The model under review builds one solid part; all positions refer to its coordinate system, in mm. A direction names the side the tool comes from. Coordinates: 2 decimals unless noted, no trailing zeros. Loops run counter-clockwise (first coordinate to the right, second up) from the corner with the lowest first, then second, coordinate; pieces in that order, holes last. Notation, with made-up numbers: M -15,79 L 0,79 A20 ccw 0,107 Z; hole C 27.5,-3 d8. An arc over 180 degrees is marked long. Use one line per item in the form item = value.
```python
from build123d import *

# Parameters (mm, degrees)
SKETCH2_W           = 118.26875
SKETCH2_H           = 122.2375
BOSS_EXTRUDE1_DEPTH = 1.5875
SKETCH3_W           = 87.78875
SKETCH3_H           = 109.5375
BOSS_EXTRUDE2_DEPTH = 12.7
SKETCH4_W           = 1.5875
SKETCH4_H           = 122.2375
BOSS_EXTRUDE3_DEPTH = 13.97
SKETCH5_W           = 87.78875
SKETCH5_H           = 9.551675444
SKETCH5_H_2         = 9.580916999
CUT_EXTRUDE1_DEPTH  = 2.5875


with BuildPart() as part:
    # Sketch2 → Boss-Extrude1 (new body)
    with BuildSketch(Plane(origin=(0, 0, 0), x_dir=(1, 0, 0), z_dir=(0, 1, 0))):
        with Locations((59.134375, 61.11875)):
            Rectangle(SKETCH2_W, SKETCH2_H)
    extrude(amount=BOSS_EXTRUDE1_DEPTH)

    # Sketch3 → Boss-Extrude2 (add)
    with BuildSketch(Plane(origin=(0, 1.5875, 0), x_dir=(1, 0, 0), z_dir=(0, 1, 0))):
        with Locations((59.134375, 61.11875)):
            Rectangle(SKETCH3_W, SKETCH3_H)
    extrude(amount=BOSS_EXTRUDE2_DEPTH)

    # Sketch4 → Boss-Extrude3 (add)
    with BuildSketch(Plane(origin=(0, 1.5875, 0), x_dir=(1, 0, 0), z_dir=(0, 1, 0))):
        with Locations((14.44625, 61.11875)):
            Rectangle(SKETCH4_W, SKETCH4_H)
        with Locations((103.8225, 61.11875)):
            Rectangle(SKETCH4_W, SKETCH4_H)
    extrude(amount=BOSS_EXTRUDE3_DEPTH)

    # Sketch5 → Cut-Extrude1 (cut, through all)
    with BuildSketch(Plane(origin=(0, 1.5875, 0), x_dir=(1, 0, 0), z_dir=(0, 1, 0))):
        with BuildLine():
            Line((-8.73125, 111.7854), (8.73125, 111.7854))
            ThreePointArc((8.73125, 111.7854), (10.97915, 109.5375), (8.73125, 107.2896))
            Line((8.73125, 107.2896), (-8.73125, 107.2896))
            ThreePointArc((-8.73125, 107.2896), (-10.97915, 109.5375), (-8.73125, 111.7854))
        make_face()
        with BuildLine():
            Line((111.91875, 111.7854), (129.38125, 111.7854))
            ThreePointArc((129.38125, 111.7854), (131.62915, 109.5375), (129.38125, 107.2896))
            Line((129.38125, 107.2896), (111.91875, 107.2896))
            ThreePointArc((111.91875, 107.2896), (109.67085, 109.5375), (111.91875, 111.7854))
        make_face()
        with BuildLine():
            Line((111.91875, 10.1854), (129.38125, 10.1854))
            ThreePointArc((129.38125, 10.1854), (131.62915, 7.9375), (129.38125, 5.6896))
            Line((129.38125, 5.6896), (111.91875, 5.6896))
            ThreePointArc((111.91875, 5.6896), (109.67085, 7.9375), (111.91875, 10.1854))
        make_face()
        with BuildLine():
            Line((-8.73125, 10.1854), (8.73125, 10.1854))
            ThreePointArc((8.73125, 10.1854), (10.97915, 7.9375), (8.73125, 5.6896))
            Line((8.73125, 5.6896), (-8.73125, 5.6896))
            ThreePointArc((-8.73125, 5.6896), (-10.97915, 7.9375), (-8.73125, 10.1854))
        make_face()
        with Locations((59.134375, 120.663337722)):
            Rectangle(SKETCH5_W, SKETCH5_H)
        with Locations((59.134375, 1.559541501)):
            Rectangle(SKETCH5_W, SKETCH5_H_2)
    extrude(amount=-CUT_EXTRUDE1_DEPTH, mode=Mode.SUBTRACT)


solid = part.part
```
1. Add section B-B (z = -26.5). State the section outline as (x, y) points, then the cut area to 3 significant figures.
Response values:
outline = M 0,0 L 118.27,0 L 118.27,1.59 L 104.62,1.59 L 104.62,15.56 L 103.03,15.56 L 103.03,14.29 L 15.24,14.29 L 15.24,15.56 L 13.65,15.56 L 13.65,1.59 L 0,1.59 Z
area = 1,350 mm^2
2. The part is to be moulded in two halves that separate along X. For faces 4 (the face through (58, 0, -62)), 5 (the face through (13.652, 8, -60)), 6 (the face through (59, 7, -6.35)), say which applies: pulls with the +X half, pulls with the -X half, needs draft (parallel to the pull), parting line crosses it, or undercut.
Response values:
face_4 = needs draft
face_5 = pulls with the -X half
face_6 = undercut
3. Add section C-C (x = 80.5). State the section outline as (y, z) points, then the cut area to 3 significant figures.
Response values:
outline = M 0,-115.89 L 14.29,-115.89 L 14.29,-6.35 L 0,-6.35 Z
area = 1,570 mm^2
4. Add section A-A (y = 12.25). State the section outline as (x, z) points, then the cut area to 3 significant figures.
Response values:
outline = M 13.65,-122.24 L 15.24,-122.24 L 15.24,-115.89 L 103.03,-115.89 L 103.03,-122.24 L 104.62,-122.24 L 104.62,0 L 103.03,0 L 103.03,-6.35 L 15.24,-6.35 L 15.24,0 L 13.65,0 Z
area = 10,000 mm^2
5. Machinability: for faces 1 (the face through (59, 14.288, -62)), 2 (the face through (15.24, 15, -61)), 3 (the face through (104.616, 8, -60)), which of the approach directions +Z, -Z, +X, -X, +Y, -Y give a long, thin tool a straight path to every point of the face, cutting with its end or side? Answer none if there is none.
Response values:
face_1 = +Z, -Z, +Y
face_2 = +Y
face_3 = +Z, -Z, +X, +Y
6. Insertion check: P1, Ø12, axis at x = 60, z = -48, coming from the +Y side; P2, Ø8, axis at x = 71, y = 2, coming from the -Z side; P3, Ø7, axis at x = 112, z = -41.5, coming from the +Y side. Each pin has a flat end and moves straight along its axis. Give the tip position at first contact, or say it passes through.
Response values:
P1 = 14.29
P2 = -115.89
P3 = 1.59
7. Wall thickness on line 1 along X through (y, z) = (15.25, -61.5); line 2 along Y through (x, z) = (97.5, -14); line 3 along Z through (x, y) = (18, 3.5): over which ranges is each line inside the solid? List them lowest first. Write a range as from..to.
Response values:
line_1 = 13.65..15.24, 103.03..104.62
line_2 = 0..14.29
line_3 = -115.89..-6.35
